Verification items for the finished model (mm, model axes). Face numbers are marked on the shaded views. A direction names the side the tool comes from. Give positions to 0.01 mm unless a question says otherwise; leave off trailing zeros. Loops run counter-clockwise (first coordinate to the right, second up) from the corner with the lowest first, then second, coordinate; pieces in that order, holes last. Notation, with made-up numbers: (28, 26) -> (53, 26) arc R22 ccw to (53, 61) -> close; hole circle Ø11 at (-26.75, 77.25). An arc over 180 degrees is marked (long way). Answer in a Markdown table with one row per item. Add a question column.
Q1. Section check B-B on z = 53. Enter the section's corners in (x, y), and give its area (3 significant figures).
Q2. Section check A-A on x = 47. Enter the section's corners in (y, z).
Q3. Release check for a two-part mould opening along Y. For the marked faces 3, 4 and 5 record: pulls with the +Y half, pulls with the -Y half, needs draft (parallel to the pull), parting line crosses it, or undercut.
Q4. Material ranges on probe 1 along Y at (x, z) = (8, -164); probe 2 along Z at (x, y) = (84, 73); probe 3 along X at (y, z) = (347, 121), recorded low to high.
Q5. Section check C-C on y = 241.5. Enter the section's corners in (x, z), and give its area (3 significant figures).
Q6. Gauge pin test, flat end, axial feed: P1, Ø5, axis at y = 114, z = 5, coming from the +X side. Record the tip position at first contact, or that the pin passes through.
Q7. Set-up check for the marked faces 1 and 2: record each of +Z, -Z, +X, -X, +Y, -Y from which the full face is reachable in a straight line by a thin tool's end or side.
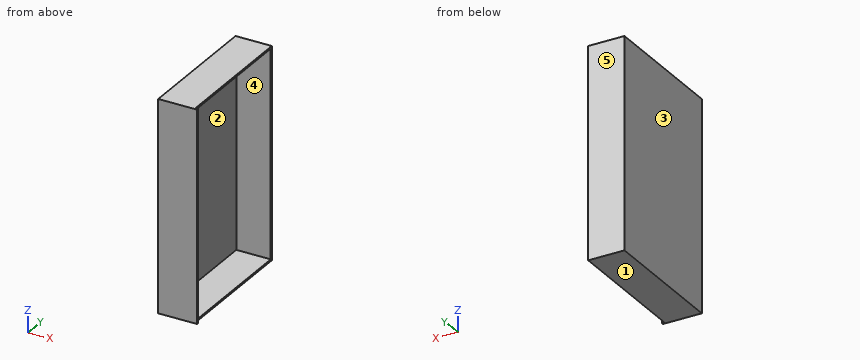
Autodesk Inventor part; units mm, degrees
ref_plane "YZ Plane" through (0, 0, 0) normal (1, 0, 0) x (0, 1, 0)
ref_plane "XZ Plane" through (0, 0, 0) normal (0, 1, 0) x (-1, 0, 0)
ref_plane "XY Plane" through (0, 0, 0) normal (0, 0, 1) x (1, 0, 0)
sketch "스케치1" plane through (0, 0, 0) normal (1, 0, 0) x (0, 1, 0)
  line L0 (367, 290) -> (0, 290)
  line L1 (0, 290) -> (0, -290)
  line L2 (0, -290) -> (367, -290)
  line L3 (367, -290) -> (367, 290)
  line L4 (362, 285) -> (5, 285)
  line L5 (5, 290) -> (5, -290)
  line L6 (5, -285) -> (362, -285)
  line L7 (362, -285) -> (362, 285)
  point P0 (0, 0)
  point P1 (0, 0)
  dimension "d0" = 367
  dimension "d1" = 580
  dimension "d2" = 5
extrude "돌출1" add sketch "스케치1" along normal blind 100 contours L3 L2 L5 L6 L7 L4 L0
extrude "돌출2" add sketch "스케치1" along normal blind 107 contours L5 L2 L1 L0
extrude "돌출3" add sketch "스케치1" along normal blind 5 contours L4 L7 L6 L5
properties part number "monitor_case" material "ABS 플라스틱"
Taken from the geometry:
| question | item | result |
|---|---|---|
| 1 | outline | (0, 0) -> (107, 0) -> (107, 5) -> (5, 5) -> (5, 362) -> (100, 362) -> (100, 367) -> (0, 367) -> close |
| 1 | area | 2,820 mm² |
| 2 | outline | (0, -290) -> (367, -290) -> (367, 290) -> (0, 290) -> close; hole (5, -285) -> (362, -285) -> (362, 285) -> (5, 285) -> close |
| 3 | face 3 | needs draft |
| 3 | face 4 | undercut |
| 3 | face 5 | pulls with the +Y half |
| 4 | probe 1 | y = 0 to 5, 362 to 367 |
| 4 | probe 2 | z = -290 to -285, 285 to 290 |
| 4 | probe 3 | x = 0 to 5 |
| 5 | outline | (0, -290) -> (100, -290) -> (100, -285) -> (5, -285) -> (5, 285) -> (100, 285) -> (100, 290) -> (0, 290) -> close |
| 5 | area | 3,850 mm² |
| 6 | P1 | stops at x = 5 |
| 7 | face 1 | -Z, +X, -X, +Y, -Y |
| 7 | face 2 | +X |
